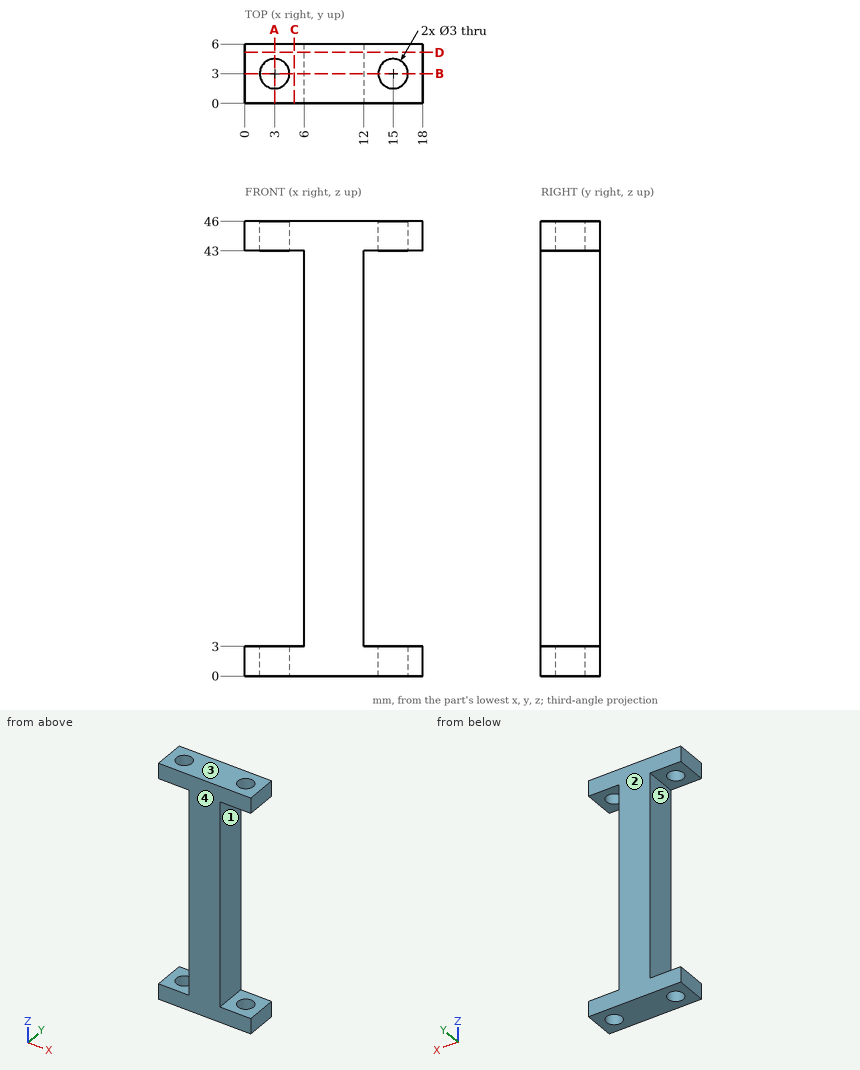
Geometry: see drawing. Coordinates: mm, zero at the bounding-box minimum. A direction names the side the tool comes from. Coordinates: 2 decimals unless noted, no trailing zeros. Write each loop counter-clockwise with the first axis right and the second up, starting at its lowest first coordinate (ties: lowest second). Pieces come first, ordered by that corner, then holes. Notation, with made-up numbers: M -10.5,36.5 L 31.5,36.5 A25 cw 31.5,59.5 Z; hole C -24,61.25 d7. An arc over 180 degrees is marked long. Answer as a JSON object with one key per item and string values.
1. Cut plane B-B on y = 3. Output: boundary loops of the cut face in (x, z).
Evaluation:
{"outline": "M 0,0 L 1.5,0 L 1.5,3 L 0,3 Z; M 0,43 L 1.5,43 L 1.5,46 L 0,46 Z; M 4.5,0 L 13.5,0 L 13.5,3 L 12,3 L 12,43 L 13.5,43 L 13.5,46 L 4.5,46 L 4.5,43 L 6,43 L 6,3 L 4.5,3 Z; M 16.5,0 L 18,0 L 18,3 L 16.5,3 Z; M 16.5,43 L 18,43 L 18,46 L 16.5,46 Z"}
2. Ray query, L1, parallel to Y at x = 3, z = 2.15; L2, parallel to Z at x = 5.25, y = 0.45; L3, parallel to X at y = 1.9, z = 43.5. Return the intervals inside material, ascending.
Evaluation:
{"L1": "0 to 1.5, 4.5 to 6", "L2": "0 to 3, 43 to 46", "L3": "0 to 1.98, 4.02 to 13.98, 16.02 to 18"}
3. Draft query along Z for the marked faces 3, 4 and 5. Return one class per face: released by +Z, released by -Z, zero draft, split by the parting line, or undercut.
Evaluation:
{"face 3": "released by +Z", "face 4": "zero draft", "face 5": "undercut"}
4. Access query for the marked faces 1 and 2. Directions: +Z, -Z, +X, -X, +Y, -Y. A direction counts if a zero-diameter tool reaches every point of the face in a straight line with its end or side. Return the directions, or none.
Evaluation:
{"face 1": "+X, +Y, -Y", "face 2": "+Z, -Z, +X, -X, +Y"}
5. Cut plane D-D on y = 5.15. Output: boundary loops of the cut face in (x, z), plus the area to 3 significant figures.
Evaluation:
{"outline": "M 0,0 L 18,0 L 18,3 L 12,3 L 12,43 L 18,43 L 18,46 L 0,46 L 0,43 L 6,43 L 6,3 L 0,3 Z", "area": "348 mm^2"}
6. Cut plane C-C on x = 5. Output: boundary loops of the cut face in (y, z), plus the area to 3 significant figures.
Evaluation:
{"outline": "M 0,0 L 6,0 L 6,3 L 0,3 Z; M 0,43 L 6,43 L 6,46 L 0,46 Z", "area": "36.0 mm^2"}
7. Contact query for flat-ended pins moving along their axis: P1, Ø2, axis at y = 2.5, z = 21, coming from the +X side; P2, Ø3, axis at y = 2.5, z = 9, coming from the -X side. Output: stop coordinate, or through.
Evaluation:
{"P1": "x = 12", "P2": "x = 6"}
8. Cut plane A-A on x = 3. Output: boundary loops of the cut face in (y, z).
Evaluation:
{"outline": "M 0,0 L 1.5,0 L 1.5,3 L 0,3 Z; M 0,43 L 1.5,43 L 1.5,46 L 0,46 Z; M 4.5,0 L 6,0 L 6,3 L 4.5,3 Z; M 4.5,43 L 6,43 L 6,46 L 4.5,46 Z"}
